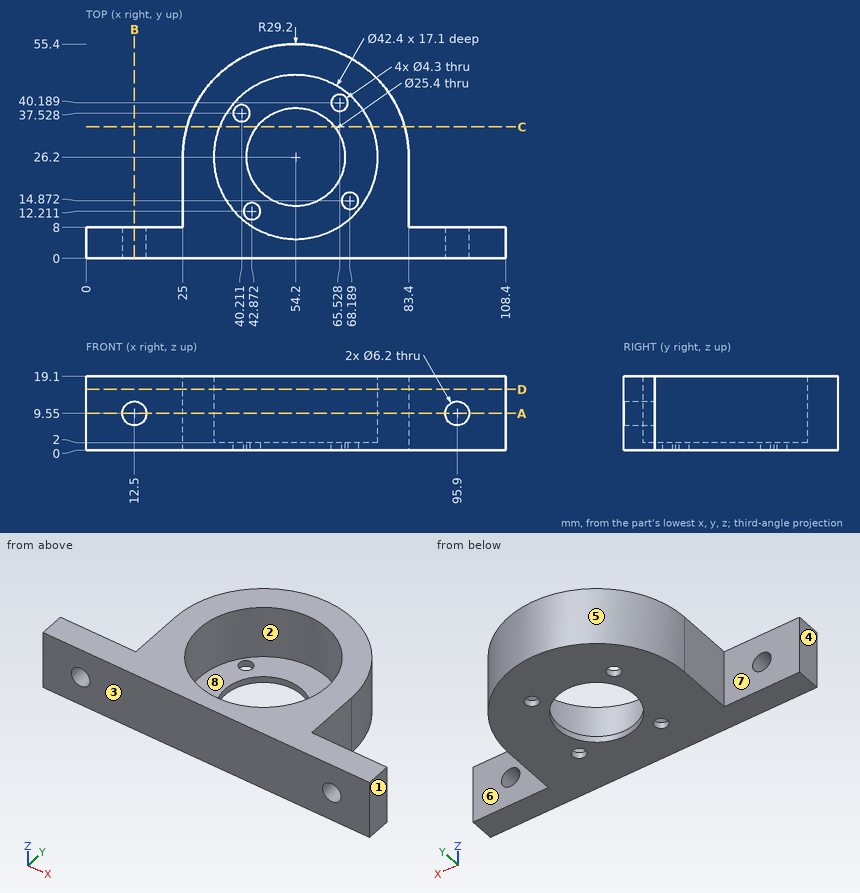
Input: dimensioned drawing with shaded views. Units: mm. Origin: part minimum x, y, z. A direction names the side the tool comes from. Coordinates: 2 decimals unless noted, no trailing zeros. Loops run counter-clockwise (first coordinate to the right, second up) from the corner with the lowest first, then second, coordinate; pieces in that order, holes last. Notation, with made-up numbers: M -23,19 L 22,19 A11 ccw 22,26 Z; hole C -34,33.25 d10. An arc over 180 degrees is marked long. Use a Markdown table: item, result. Add a question column.
1) Section C-C, the plane y = 34. Return the cut outline in (x, z).
2) Set-up query: the marked faces 4, 5, 6, 7 and 8. Return all of +Z, -Z, +X, -X, +Y, -Y with unobstructed straight access to the full face (end or side cutting, diameter ignored); none if empty.
3) Section D-D, the plane z = 15.75. Return the cut outline in (x, y), plus the area to 3 significant figures.
4) Pin query (flat end, axial travel): P1, Ø5, axis at x = 65.53, y = 40.19, coming from the +Z side; P2, Ø8, axis at y = 13.5, z = 17, coming from the -X side; P3, Ø6, axis at x = 63, z = 11.5, coming from the +Y side; P4, Ø10, axis at x = 22.5, z = 9.5, coming from the -Y side. Return the tip coordinate at first contact, or that it passes through.
5) Draft query along Y for the marked faces 1, 2 and 3. Return one class per face: +Y half, -Y half, draft (parallel to the pull), parting line (faces both ways), or undercut.
6) Line query: L1, parallel to Y at x = 54.2, z = 0.65; L2, parallel to X at y = 26.2, z = 0.5; L3, parallel to Y at x = 54.2, z = 7.25. Output: solid intervals per line, ascending. Write a range as from..to.
7) Section B-B, the plane x = 12.5. Return the cut outline in (y, z).
8) Section A-A, the plane z = 9.55. Return the cut outline in (x, y).
Answer below:
| question | item | result |
|---|---|---|
| 1 | outline | M 26.06,0 L 44.18,0 L 44.18,2 L 34.49,2 L 34.49,19.1 L 26.06,19.1 Z; M 64.22,0 L 82.34,0 L 82.34,19.1 L 73.91,19.1 L 73.91,2 L 64.22,2 Z |
| 2 | face 4 | +Z, -Z, -X, +Y, -Y |
| 2 | face 5 | +Z, -Z, +Y |
| 2 | face 6 | +Z, -Z, +X, +Y |
| 2 | face 7 | +Z, -Z, -X, +Y |
| 2 | face 8 | +Z |
| 3 | outline | M 0,0 L 108.4,0 L 108.4,8 L 83.4,8 L 83.4,26.2 A29.2 ccw 25,26.2 L 25,8 L 0,8 Z; hole C 54.2,26.2 d42.4 |
| 3 | area | 1,860 mm2 |
| 4 | P1 | z = 2 |
| 4 | P2 | x = 25 |
| 4 | P3 | y = 54.82 |
| 4 | P4 | y = 0 |
| 5 | face 1 | draft |
| 5 | face 2 | undercut |
| 5 | face 3 | -Y half |
| 6 | L1 | 0..13.5, 38.9..55.4 |
| 6 | L2 | 25..41.5, 66.9..83.4 |
| 6 | L3 | 0..5, 47.4..55.4 |
| 7 | outline | M 0,0 L 8,0 L 8,6.45 L 0,6.45 Z; M 0,12.65 L 8,12.65 L 8,19.1 L 0,19.1 Z |
| 8 | outline | M 0,0 L 9.4,0 L 9.4,8 L 0,8 Z; M 15.6,0 L 92.8,0 L 92.8,8 L 83.4,8 L 83.4,26.2 A29.2 ccw 25,26.2 L 25,8 L 15.6,8 Z; M 99,0 L 108.4,0 L 108.4,8 L 99,8 Z; hole C 54.2,26.2 d42.4 |
